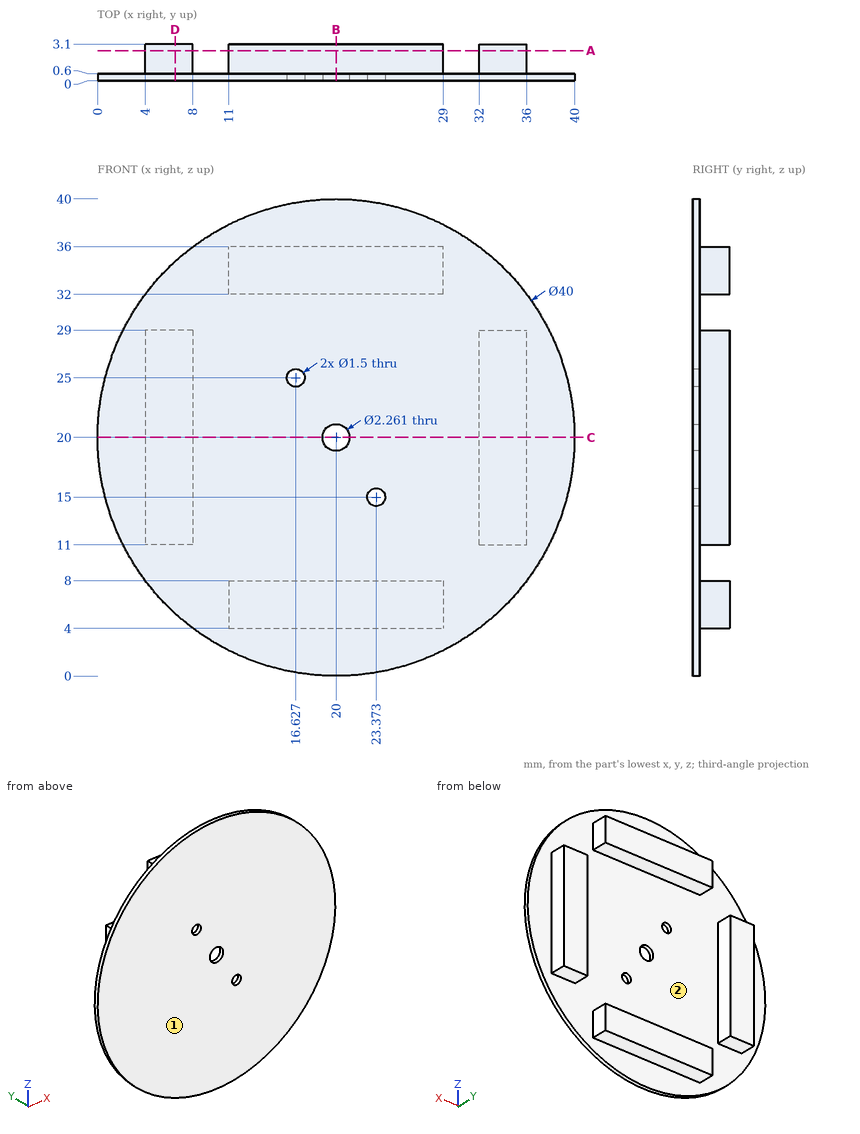
Part print with two shaded views. Sizes in mm from the minimum x, y, z corner. Round coordinates to 2 decimals unless told otherwise and drop trailing zeros. Order: outer loops, then holes, each group sorted by start corner. A loop starts at its lowest first (then second) coordinate and runs counter-clockwise, first axis right, second up. Notation, with made-up numbers: M 37,-25.75 L 46,-25.75 A19 ccw 46,-15.75 Z; hole C 71.5,39.5 d5. An arc over 180 degrees is marked long. Answer in a Markdown table with one row per item. Add a question column.
Q1. Wall check: L1, parallel to X at y = 1.6, z = 18; L2, parallel to X at y = 0.2, z = 20. Give the ranges that are in metal, low to high. Write a range as from..to.
Q2. Cut at A-A on y = 2.55. Give the cut face in (x, z).
Q3. Cut at C-C on z = 20. Give the cut face in (x, y).
Q4. Pin check, flat tips, straight feed: pin 1 (1.2 mm diameter, centred on x = 24, y = 1.5, fed in from -Z); pin 2 (10 mm diameter, centred on x = 13.5, z = 6.5, fed in from -Y); pin 3 (1 mm diameter, centred on x = 12, y = 1, fed in from -Z); pin 4 (1 mm diameter, centred on y = 1.5, z = 13, fed in from +X). Stop position of each tip, or through.
Q5. Mould opens along X. For the marked faces 1 and 2 say: +X half, -X half, draft (parallel to the pull), parting line (faces both ways), or undercut.
Q6. Cut at B-B on x = 20. Give the cut face in (y, z).
Q7. Cut at D-D on x = 6.5. Give the cut face in (y, z).
Established:
| question | item | result |
|---|---|---|
| 1 | L1 | x = 4..8, 32..36 |
| 1 | L2 | x = 0..18.87, 21.13..40 |
| 2 | outline | M 4,11 L 8,11 L 8,29 L 4,29 Z; M 11,4 L 29,4 L 29,8 L 11,8 Z; M 11,32 L 29,32 L 29,36 L 11,36 Z; M 32,11 L 36,11 L 36,29 L 32,29 Z |
| 3 | outline | M 0,0 L 18.87,0 L 18.87,0.6 L 8,0.6 L 8,3.1 L 4,3.1 L 4,0.6 L 0,0.6 Z; M 21.13,0 L 40,0 L 40,0.6 L 36,0.6 L 36,3.1 L 32,3.1 L 32,0.6 L 21.13,0.6 Z |
| 4 | pin 1 | stops at z = 4 |
| 4 | pin 2 | stops at y = 0 |
| 4 | pin 3 | stops at z = 1.54 |
| 4 | pin 4 | stops at x = 36 |
| 5 | face 1 | draft |
| 5 | face 2 | undercut |
| 6 | outline | M 0,0 L 0.6,0 L 0.6,4 L 3.1,4 L 3.1,8 L 0.6,8 L 0.6,18.87 L 0,18.87 Z; M 0,21.13 L 0.6,21.13 L 0.6,32 L 3.1,32 L 3.1,36 L 0.6,36 L 0.6,40 L 0,40 Z |
| 7 | outline | M 0,5.24 L 0.6,5.24 L 0.6,11 L 3.1,11 L 3.1,29 L 0.6,29 L 0.6,34.76 L 0,34.76 Z |
